from build123d import *

# Parameters (mm, degrees)
SKETCH1_W             = 10
SKETCH1_H             = 8
BOSS_EXTRUDE1_DEPTH   = 21
BOSS_EXTRUDE1_2_DEPTH = 21
BOSS_EXTRUDE2_DEPTH   = 5


with BuildPart() as part:
    # Sketch1 → Boss-Extrude1 (new body)
    with BuildSketch(Plane(origin=(0, 0, 0), x_dir=(1, 0, 0), z_dir=(0, 1, 0))):
        with Locations((-60.425, 0)):
            Rectangle(SKETCH1_W, SKETCH1_H)
    extrude(amount=BOSS_EXTRUDE1_DEPTH)



with BuildPart() as body_2:
    # Sketch1 → Boss-Extrude1 2 (new body)
    with BuildSketch(Plane(origin=(0, 0, 0), x_dir=(1, 0, 0), z_dir=(0, 1, 0))):
        with Locations((60.425, 0)):
            Rectangle(SKETCH1_W, SKETCH1_H)
    extrude(amount=BOSS_EXTRUDE1_2_DEPTH)


with BuildPart() as part_1:
    add(part.part)

    add(body_2.part)  # Boss-Extrude2 merges body 2
    # Sketch2 → Boss-Extrude2 (add)
    with BuildSketch(Plane(origin=(0, 21, 0), x_dir=(1, 0, 0), z_dir=(0, 1, 0))):
        with BuildLine():
            Line((-21.75, 21.75), (21.75, 21.75))
            Line((21.75, 21.75), (51.042007296, 21.75))
            ThreePointArc((51.042007296, 21.75), (54.826187522, 20.725336286), (57.576364504, 17.931328005))
            Line((57.576364504, 17.931328005), (65.425, 4))
            Line((65.425, 4), (65.425, -4))
            Line((65.425, -4), (34.770583875, -4))
            ThreePointArc((34.770583875, -4), (31.010557787, -5.010608363), (28.263842049, -7.770078981))
            Line((28.263842049, -7.770078981), (20.25, -21.75))
            Line((20.25, -21.75), (-20.25, -21.75))
            Line((-20.25, -21.75), (-28.263842049, -7.770078981))
            ThreePointArc((-28.263842049, -7.770078981), (-31.010557787, -5.010608363), (-34.770583875, -4))
            Line((-34.770583875, -4), (-65.425, -4))
            Line((-65.425, -4), (-65.425, 4))
            Line((-65.425, 4), (-57.576364504, 17.931328005))
            ThreePointArc((-57.576364504, 17.931328005), (-54.826187522, 20.725336286), (-51.042007296, 21.75))
            Line((-51.042007296, 21.75), (-21.75, 21.75))
        make_face()
    extrude(amount=BOSS_EXTRUDE2_DEPTH)


solid = part_1.part
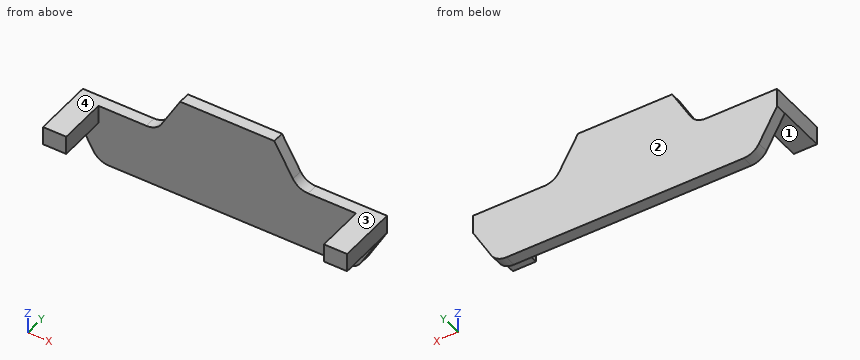
Could you check a few things on this model? Use its own coordinates, in mm. Face numbers are marked on the shaded views. A direction names the side the tool comes from. Give positions to 0.01 mm unless a question says otherwise; leave off trailing zeros. Order: outer loops, then holes, each group sorted by start corner. A loop starts at its lowest first (then second) coordinate and runs counter-clockwise, first axis right, second up. Notation, with made-up numbers: (-1.5, -29) -> (14.5, -29) arc R35 ccw to (14.5, 4) -> close; hole circle Ø11 at (-7, 8.25). An arc over 180 degrees is marked (long way). Answer in a Markdown table with one row per item. Add a question column.
Item 1: Please list where these lines run through material, in increasing order: probe 1 along X at (y, z) = (4.5, 3.5) (3 decimals); probe 2 along Y at (x, z) = (13.5, -2.5); probe 3 along Z at (x, y) = (43, 25).
Item 2: Imagine slicing it at B-B (z = -1.5). List the corners of the cut face in (x, y) for me (3 decimals).
Item 3: For the marked faces 1, 2, 3 and 4, which set-ups out of +Z, -Z, +X, -X, +Y, -Y let a thin tool reach every point of the face, with its end or its side?
Item 4: Imagine slicing it at D-D (x = 41.5). List the corners of the cut face in (y, z) for me.
Item 5: Imagine slicing it at C-C (y = 22.5). List the corners of the cut face in (x, z) for me (3 decimals), and give its area (3 significant figures).
Item 6: Imagine slicing it at A-A (y = 3.5). List the corners of the cut face in (x, z) for me (3 decimals).
Item 7: I'm going to push flat-ended pins straight in: P1, Ø4, axis at x = 0, z = 12.5, coming from the -Y side; P2, Ø3, axis at x = 62.5, y = 11, coming from the -Z side. Where does each tip first touch, or does it pass through?
Result:
| question | item | result |
|---|---|---|
| 1 | probe 1 | -65.425 to -55.425, 55.425 to 65.425 |
| 1 | probe 2 | 21 to 26 |
| 1 | probe 3 | -21.75 to 4 |
| 2 | outline | (-65.425, 0) -> (-55.425, 0) -> (-55.425, 21) -> (55.425, 21) -> (55.425, 0) -> (65.425, 0) -> (65.425, 26) -> (-65.425, 26) -> close |
| 3 | face 1 | -Z, +X, -X, -Y |
| 3 | face 2 | +Z, -Z, +X, -X, +Y |
| 3 | face 3 | +Z, +X, +Y, -Y |
| 3 | face 4 | +Z, -X, +Y, -Y |
| 4 | outline | (21, -21.75) -> (26, -21.75) -> (26, 4) -> (21, 4) -> close |
| 5 | outline | (-65.425, -4) -> (-57.576, -17.931) arc R7.5 ccw to (-51.042, -21.75) -> (51.042, -21.75) arc R7.5 ccw to (57.576, -17.931) -> (65.425, -4) -> (65.425, 4) -> (34.771, 4) arc R7.5 cw to (28.264, 7.77) -> (20.25, 21.75) -> (-20.25, 21.75) -> (-28.264, 7.77) arc R7.5 cw to (-34.771, 4) -> (-65.425, 4) -> close |
| 5 | area | 4,090 mm2 |
| 6 | outline | (-65.425, -4) -> (-55.425, -4) -> (-55.425, 4) -> (-65.425, 4) -> close; (55.425, -4) -> (65.425, -4) -> (65.425, 4) -> (55.425, 4) -> close |
| 7 | P1 | y = 21 |
| 7 | P2 | z = -4 |
